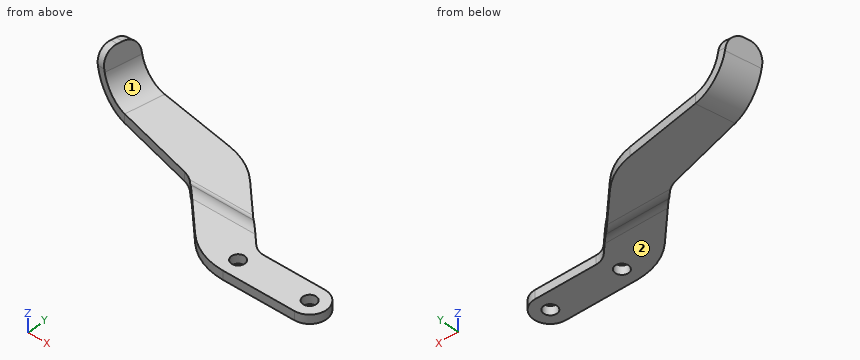
from build123d import *

# Parameters (mm, degrees)
BASE_EXTRUDE_DEPTH      = 3.175
CUT_EXTRUDE1_DEPTH      = 101.324569797
CUT_EXTRUDE1_DEPTH_BACK = 101.324569797
CUT_EXTRUDE2_DEPTH      = 101.3245698
SKETCH4_R               = 2.38125
CUT_EXTRUDE3_DEPTH      = 101.47517694
BOSS_EXTRUDE1_REACH     = 102.663
FILLET4_R               = 5.334


with BuildPart() as part:
    # Sketch1 → Base-Extrude (new, symmetric)
    with BuildSketch(Plane.XY):
        with BuildLine():
            Line((0, 6), (-21.525, 6))
            ThreePointArc((-21.525, 6), (-23.955039796, 6.483364969), (-26.015128061, 7.859871939))
            Line((-26.015128061, 7.859871939), (-47.883548214, 29.728292093))
            ThreePointArc((-47.883548214, 29.728292093), (-54.11564568, 34.297855014), (-61.433396744, 36.781896777))
            Line((-61.433396744, 36.781896777), (-88.9, 41.625))
            Line((-88.9, 41.625), (-91.226630185, 28.43002453))
            Line((-91.226630185, 28.43002453), (-63.378809052, 20.968223346))
            ThreePointArc((-63.378809052, 20.968223346), (-61.081560456, 20.016671822), (-59.108868366, 18.502971942))
            Line((-59.108868366, 18.502971942), (-41.115448212, 0.509551788))
            ThreePointArc((-41.115448212, 0.509551788), (-33.905139284, -4.30822261), (-25.4, -6))
            Line((-25.4, -6), (0, -6))
            ThreePointArc((0, -6), (6, 0), (0, 6))
        make_face()
    extrude(amount=BASE_EXTRUDE_DEPTH, both=True)

    # Sketch2 → Cut-Extrude1 (cut, two sides)
    with BuildSketch(Plane(origin=(0, 0, 0), x_dir=(0, 0, -1), z_dir=(1, 0, 0))) as cut_extrude1_sk:
        with BuildLine():
            Line((109.267936785, -6), (3.175, -6))
            Line((3.175, -6), (0, -6))
            Line((0, -6), (0, 10.999739587))
            ThreePointArc((0, 10.999739587), (0.410118898, 13.244803618), (1.5875, 15.199869794))
            ThreePointArc((1.5875, 15.199869794), (2.764881102, 17.15493597), (3.175, 19.4))
            Line((3.175, 19.4), (3.175, 125.492936785))
            Line((3.175, 125.492936785), (168.312411522, 258.731370649))
            Line((168.312411522, 258.731370649), (274.405348307, 127.238433864))
            Line((274.405348307, 127.238433864), (109.267936785, -6))
        make_face()
    extrude(amount=CUT_EXTRUDE1_DEPTH, mode=Mode.SUBTRACT)
    extrude(cut_extrude1_sk.sketch, amount=-CUT_EXTRUDE1_DEPTH_BACK, mode=Mode.SUBTRACT)

    # Sketch3 → Cut-Extrude2 (cut, through all)
    with BuildSketch(Plane(origin=(0, 0, 0), x_dir=(0, 0, -1), z_dir=(1, 0, 0))):
        with BuildLine():
            Line((0, 19.4), (0, 41.625))
            Line((0, 41.625), (-3.175, 41.625))
            Line((-3.175, 41.625), (-3.175, 10.999739587))
            ThreePointArc((-3.175, 10.999739587), (-2.559821652, 14.367335633), (-0.79375, 17.299934897))
            ThreePointArc((-0.79375, 17.299934897), (-0.205059449, 18.277467985), (0, 19.4))
        make_face()
    extrude(amount=-CUT_EXTRUDE2_DEPTH, mode=Mode.SUBTRACT)

    # Sketch4 → Cut-Extrude3 (cut, through all)
    with BuildSketch(Plane.XY.offset(3.175)):
        Circle(SKETCH4_R)
        with Locations((-25.4, 0)):
            Circle(SKETCH4_R)
    extrude(amount=-CUT_EXTRUDE3_DEPTH, mode=Mode.SUBTRACT)

    # Boss-Extrude1: up to this plane
    boss_extrude1_end = Plane(origin=(-63.378809052, 20.968223346, 3.175), z_dir=(-0.2588190451025212, -0.9659258262890683, 0))
    # Sketch6 → Boss-Extrude1 (add, up to the surface)
    with BuildSketch(Plane(origin=(4.437631227, 25.167057299, 0), x_dir=(-0.9848077530122081, 0.1736481776669304, 0), z_dir=(0.17364817766693036, 0.984807753012208, 0)), mode=Mode.PRIVATE) as boss_extrude1_sk1:
        with BuildLine():
            Line((94.777514638, -3.175), (94.777514638, 0))
            ThreePointArc((94.777514638, 0), (100.893829519, 2.100047584), (104.430088098, 7.51432342))
            Line((104.430088098, 7.51432342), (105.962866768, 13.571805745))
            Line((105.962866768, 13.571805745), (109.040855754, 12.792954794))
            Line((109.040855754, 12.792954794), (107.508077084, 6.73547247))
            ThreePointArc((107.508077084, 6.73547247), (102.844185029, -0.405294385), (94.777514638, -3.175))
        make_face()
    boss_extrude1_tool1 = split(extrude(boss_extrude1_sk1.sketch, amount=-BOSS_EXTRUDE1_REACH, mode=Mode.PRIVATE), bisect_by=boss_extrude1_end, keep=Keep.BOTH, mode=Mode.PRIVATE)
    add(boss_extrude1_tool1.solids().sort_by_distance((-96.950625, 43.044542, 3.972737))[0])

    # Fillet4
    fillet4_edges = [part.edges().sort_by_distance(p)[0] for p in [
        (-103.564353975, 31.735907656, 13.182380269),
        (-101.431035206, 43.834559603, 13.182380269),
    ]]
    fillet(fillet4_edges, radius=FILLET4_R)


solid = part.part
Input: part model. Units: mm. Frame: model coordinates. Face numbers are marked on the shaded views. A direction names the side the tool comes from. Round coordinates to 2 decimals unless told otherwise and drop trailing zeros. Order: outer loops, then holes, each group sorted by start corner. A loop starts at its lowest first (then second) coordinate and runs counter-clockwise, first axis right, second up.
1. Cut plane D-D, the plane y = 13. Output: boundary loops of the cut face in (x, z).
The answers:
outline: (-53.61, -0.32) - (-31.16, -0.32) - (-31.16, 2.96) - (-53.61, 2.96) - close
2. Material intervals for line 1 (Y direction, x = 0, z = 1.5); line 2 (Z direction, x = -73.5, y = 26.5) (3 decimals); line 3 (Y direction, x = -47, z = 1.25), sorted ascending.
The answers:
line 1: y = -6 to -2.38, 2.38 to 6
line 2: z = -3.175 to 0
line 3: y = 6.39 to 16.74
3. Set-up query: the marked faces 1 and 2. Return all of +Z, -Z, +X, -X, +Y, -Y with unobstructed straight access to the full face (end or side cutting, diameter ignored); none if empty.
The answers:
face 1: +Z, +X, -Y
face 2: -Z, +X, -X, -Y
4. Cut plane A-A, the plane x = -1. Output: boundary loops of the cut face in (y, z) (3 decimals).
The answers:
outline: (-6, 0) - (-2.161, 0) - (-2.161, 3.175) - (-6, 3.175) - close; (2.161, 0) - (6, 0) - (6, 3.175) - (2.161, 3.175) - close
5. Pin query (flat end, axial travel): P1, Ø8, axis at y = 21.5, z = 6.5, coming from the -X side; P2, Ø1, axis at x = -10, z = 1, coming from the +Y side; P3, Ø5.5, axis at x = 0, y = 0, coming from the +Z side (3 decimals); P4, Ø12, axis at x = -45.5, y = 1.5, coming from the -Z side. Return the tip coordinate at first contact, or that it passes through.
The answers:
P1: passes through
P2: stops at y = 6
P3: stops at z = 3.175
P4: stops at z = 0
6. Cut plane C-C, the plane z = 4.5. Output: boundary loops of the cut face in (x, y), then the cut area to 3 significant figures.
The answers:
outline: (-102.81, 31.53) - (-99.3, 30.59) - (-97.1, 43.07) - (-100.66, 43.7) - close
area: 45.2 mm2
